```python
from build123d import *

# Parameters (mm, degrees)
F0_R     = 15.24
F0_R_2   = 10.16
F1_DEPTH = 101.6
F3_DEPTH = 38.1


with BuildPart() as f1:
    # F0 (on Top) → F1 (new body)
    with BuildSketch(Plane.XY):
        Circle(F0_R)
        Circle(F0_R_2, mode=Mode.SUBTRACT)
    extrude(amount=F1_DEPTH)


with BuildPart() as f3:
    # F2 (on Right) → F3 (new body, symmetric)
    with BuildSketch(Plane.YZ):
        Polygon((-8.89, 34.2392), (0, 34.2392), (8.89, 34.2392), (8.89, 38.0492), (-8.89, 38.0492), align=None)
    extrude(amount=F3_DEPTH, both=True)


with BuildPart() as f1_1:
    add(f1.part)

    # F4: cut F3
    add(f3.part, mode=Mode.SUBTRACT)


solid = f1_1.part
```
The model under review builds one solid part; all positions refer to its coordinate system, in mm. A direction names the side the tool comes from. Coordinates: 2 decimals unless noted, no trailing zeros. Write each loop counter-clockwise with the first axis right and the second up, starting at its lowest first coordinate (ties: lowest second). Pieces come first, ordered by that corner, then holes. Notation, with made-up numbers: (21, 71.5) - (61, 71.5) arc R9 ccw to (61, 87.5) - close; hole circle Ø3 at (81, 32.25). An arc over 180 degrees is marked (long way). Write item = value, one per line.
(1) For line 1 (Y direction, x = 0, z = 46); line 2 (X direction, y = 0.5, z = 58); line 3 (Y direction, x = 7, z = 16), list the stretches that pass through material, from the lowest coordinate up. Write a range as [from, to].
Result sheet:
line_1 = [-15.24, -10.16], [10.16, 15.24]
line_2 = [-15.23, -10.15], [10.15, 15.23]
line_3 = [-13.54, -7.36], [7.36, 13.54]
(2) Mouldability with a two-part tool opening along Z and no side actions: class faces 1 (the face through (11, 0, 34.239)), 2 (the face through (3, -10, 101.6)), 3 (the face through (3, -10, 0)) as pulls with the +Z half, pulls with the -Z half, needs draft (parallel to the pull), parting line crosses it, or undercut.
Result sheet:
face_1 = undercut
face_2 = pulls with the +Z half
face_3 = pulls with the -Z half
(3) For P1, Ø1.5, axis at y = 1.5, z = 55, coming from the -X side; P2, Ø3, axis at x = 8.5, z = 37, coming from the -Y side; P3, Ø1.5, axis at y = -11, z = 78, coming from the -X side, all flat-tipped, find the tip position at first contact; note any pin that passes through.
Result sheet:
P1 = -15.22
P2 = -13.54
P3 = -11.28
(4) Consider section A-A, the plane x = 0. Give the boundary of the cut face in (y, z), then the cut area to 3 significant figures.
Result sheet:
outline = (-15.24, 0) - (-10.16, 0) - (-10.16, 101.6) - (-15.24, 101.6) - close; (10.16, 0) - (15.24, 0) - (15.24, 101.6) - (10.16, 101.6) - close
area = 1,030 mm^2
(5) Machinability: for faces 4 (the face through (-3.3, -14.88, 50.09)), 5 (the face through (-11, 0, 38.049)), which of the approach directions +Z, -Z, +X, -X, +Y, -Y give a long, thin tool a straight path to every point of the face, cutting with its end or side? Answer none if there is none.
Result sheet:
face_4 = +Z, -Z
face_5 = +X, -X
(6) Consider section B-B, the plane y = 0. Give the boundary of the cut face in (x, z).
Result sheet:
outline = (-15.24, 0) - (-10.16, 0) - (-10.16, 34.24) - (-15.24, 34.24) - close; (-15.24, 38.05) - (-10.16, 38.05) - (-10.16, 101.6) - (-15.24, 101.6) - close; (10.16, 0) - (15.24, 0) - (15.24, 34.24) - (10.16, 34.24) - close; (10.16, 38.05) - (15.24, 38.05) - (15.24, 101.6) - (10.16, 101.6) - close
(7) Consider section C-C, the plane z = 44. Give the boundary of the cut face in (x, y), then the cut area to 3 significant figures.
Result sheet:
outline = circle Ø30.48 at (0, 0); hole circle Ø20.32 at (0, 0)
area = 405 mm^2
(8) Consider section D-D, the plane y = -5. Give the boundary of the cut face in (x, z), then the cut area to 3 significant figures.
Result sheet:
outline = (-14.4, 0) - (-8.84, 0) - (-8.84, 34.24) - (-14.4, 34.24) - close; (-14.4, 38.05) - (-8.84, 38.05) - (-8.84, 101.6) - (-14.4, 101.6) - close; (8.84, 0) - (14.4, 0) - (14.4, 34.24) - (8.84, 34.24) - close; (8.84, 38.05) - (14.4, 38.05) - (14.4, 101.6) - (8.84, 101.6) - close
area = 1,090 mm^2
